Check sheet for the modelled part. Datum: model origin and axes. Units: mm. A direction names the side the tool comes from. Round coordinates to 2 decimals unless told otherwise and drop trailing zeros. Write each loop counter-clockwise with the first axis right and the second up, starting at its lowest first coordinate (ties: lowest second). Pieces come first, ordered by that corner, then holes. Notation, with made-up numbers: (-6.5, -8) -> (23.5, -8) arc R19 ccw to (23.5, 29) -> close; hole circle Ø6 at (30.5, 66.25). An arc over 180 degrees is marked (long way). One line per item, written item: value.
from build123d import *

# Parameters (mm, degrees)
SKETCH_2_W      = 200
SKETCH_2_H      = 120
SKETCH_2_R      = 1.6
EXTRUDE_1_DEPTH = 5
FILLET_1_R      = 10


with BuildPart() as part:
    # 草图2 → 凸台-拉伸1 (new body)
    with BuildSketch(Plane(origin=(0, 0, 0), x_dir=(1, 0, 0), z_dir=(0, 1, 0))):
        with Locations((100, 60)):
            Rectangle(SKETCH_2_W, SKETCH_2_H)
        with Locations(Location((187, 45, 0), (0, 0, 270))):
            Circle(SKETCH_2_R, mode=Mode.SUBTRACT)
        with Locations(Location((187, 75, 0), (0, 0, 90))):
            Circle(SKETCH_2_R, mode=Mode.SUBTRACT)
        with Locations(Location((163, 45, 0), (0, 0, 270))):
            Circle(SKETCH_2_R, mode=Mode.SUBTRACT)
        with Locations(Location((163, 75, 0), (0, 0, 90))):
            Circle(SKETCH_2_R, mode=Mode.SUBTRACT)
        with Locations(Location((13, 45, 0), (0, 0, 90))):
            Circle(SKETCH_2_R, mode=Mode.SUBTRACT)
        with Locations(Location((37, 45, 0), (0, 0, 90))):
            Circle(SKETCH_2_R, mode=Mode.SUBTRACT)
        with Locations(Location((13, 75, 0), (0, 0, 270))):
            Circle(SKETCH_2_R, mode=Mode.SUBTRACT)
        with Locations(Location((37, 75, 0), (0, 0, 270))):
            Circle(SKETCH_2_R, mode=Mode.SUBTRACT)
        with Locations(Location((196, 97, 0), (0, 0, 270))):
            Circle(SKETCH_2_R, mode=Mode.SUBTRACT)
        with Locations(Location((136, 97, 0), (0, 0, 270))):
            Circle(SKETCH_2_R, mode=Mode.SUBTRACT)
        with Locations(Location((196, 23, 0), (0, 0, 90))):
            Circle(SKETCH_2_R, mode=Mode.SUBTRACT)
        with Locations(Location((136, 23, 0), (0, 0, 90))):
            Circle(SKETCH_2_R, mode=Mode.SUBTRACT)
        with Locations(Location((4, 23, 0), (0, 0, 270))):
            Circle(SKETCH_2_R, mode=Mode.SUBTRACT)
        with Locations(Location((4, 97, 0), (0, 0, 90))):
            Circle(SKETCH_2_R, mode=Mode.SUBTRACT)
        with Locations(Location((64, 23, 0), (0, 0, 270))):
            Circle(SKETCH_2_R, mode=Mode.SUBTRACT)
        with Locations(Location((64, 97, 0), (0, 0, 90))):
            Circle(SKETCH_2_R, mode=Mode.SUBTRACT)
        with BuildLine():
            Line((153.5, 115), (178.5, 115))
            ThreePointArc((178.5, 115), (183.5, 110), (178.5, 105))
            Line((178.5, 105), (153.5, 105))
            ThreePointArc((153.5, 105), (148.5, 110), (153.5, 115))
        make_face(mode=Mode.SUBTRACT)
        with BuildLine():
            Line((153.5, 5), (178.5, 5))
            ThreePointArc((178.5, 5), (183.5, 10), (178.5, 15))
            Line((178.5, 15), (153.5, 15))
            ThreePointArc((153.5, 15), (148.5, 10), (153.5, 5))
        make_face(mode=Mode.SUBTRACT)
        with BuildLine():
            Line((46.5, 115), (21.5, 115))
            ThreePointArc((21.5, 115), (16.5, 110), (21.5, 105))
            Line((21.5, 105), (46.5, 105))
            ThreePointArc((46.5, 105), (51.5, 110), (46.5, 115))
        make_face(mode=Mode.SUBTRACT)
        with BuildLine():
            Line((46.5, 5), (21.5, 5))
            ThreePointArc((21.5, 5), (16.5, 10), (21.5, 15))
            Line((21.5, 15), (46.5, 15))
            ThreePointArc((46.5, 15), (51.5, 10), (46.5, 5))
        make_face(mode=Mode.SUBTRACT)
    extrude(amount=EXTRUDE_1_DEPTH)

    # 圆角1
    fillet_1_edges = [part.edges().sort_by_distance(p)[0] for p in [
        (0, 2.5, -120),
        (200, 2.5, -120),
        (200, 2.5, 0),
        (0, 2.5, 0),
    ]]
    fillet(fillet_1_edges, radius=FILLET_1_R)


solid = part.part
Item 1: Sectioned sample at A-A (x = 49). Enter the section's corners in (y, z).
Result set:
outline: (0, -120) -> (5, -120) -> (5, -114.33) -> (0, -114.33) -> close; (0, -105.67) -> (5, -105.67) -> (5, -14.33) -> (0, -14.33) -> close; (0, -5.67) -> (5, -5.67) -> (5, 0) -> (0, 0) -> close
Item 2: Material ranges on line 1 along X through (y, z) = (2.9, -75); line 2 along Z through (x, y) = (163, 3); line 3 along Z through (x, y) = (43, 1.7), recorded low to high.
Result set:
line 1: 0 to 11.4, 14.6 to 35.4, 38.6 to 161.4, 164.6 to 185.4, 188.6 to 200
line 2: -120 to -115, -105 to -76.6, -73.4 to -46.6, -43.4 to -15, -5 to 0
line 3: -120 to -115, -105 to -15, -5 to 0
Item 3: Release check for a two-part mould opening along X. For faces 3 (the cylindrical face through (51.5, 2.5, -10.1)), 4 (the flat face through (200, 2, -59)), 5 (the cylindrical face through (2.85, 2.54, -116.99)) record: pulls with the +X half, pulls with the -X half, needs draft (parallel to the pull), parting line crosses it, or undercut.
Result set:
face 3: undercut
face 4: pulls with the +X half
face 5: pulls with the -X half
Item 4: Sectioned sample at B-B (y = 1.05). State how many separate pieces and enclosed holes the cut face has, then the cut area to 3 significant figures.
Result set:
separate pieces: 1
enclosed holes: 20
area: 22,500 mm^2
Item 5: Depth check by flat-ended pin: pin 1 (3 mm diameter, centred on x = 37, z = -75, fed in from +Y). Enter the tip coordinate at first touch or a pass-through.
Result set:
pin 1: through
Item 6: Tool access check on faces 1 (the flat face through (99, 2, 0)), 2 (the cylindrical face through (183.5, 2.5, -9.9)). Record the directions out of +Z, -Z, +X, -X, +Y, -Y that give a thin tool (end or side, any length) a straight path to the whole face; none if there is none.
Result set:
face 1: +Z, +X, -X, +Y, -Y
face 2: +Y, -Y
